Here's how the part is built. I have some questions about the finished solid (model axes, mm). A direction names the side the tool comes from. Round coordinates to 2 decimals unless told otherwise and drop trailing zeros. Loops run counter-clockwise (first coordinate to the right, second up) from the corner with the lowest first, then second, coordinate; pieces in that order, holes last. Notation, with made-up numbers: M 67.5,50 L 104.5,50 A25 cw 104.5,64 Z; hole C 63.25,-24 d11. An arc over 180 degrees is marked long. Answer as CSV lines item,"result".
```python
from build123d import *

# Parameters (mm, degrees)
SKETCH1_W           = 92.25
SKETCH1_H           = 72
SKETCH1_R           = 15
BOSS_EXTRUDE1_DEPTH = 36
BOSS_EXTRUDE2_START = -16
SKETCH1_3_R         = 36
SKETCH1_3_R_2       = 15
BOSS_EXTRUDE2_DEPTH = 16
SKETCH2_R           = 12
BOSS_EXTRUDE3_DEPTH = 28.575


with BuildPart() as part:
    # Sketch1 → Boss-Extrude1 (new body)
    with BuildSketch(Plane(origin=(0, 0, 0), x_dir=(1, 0, 0), z_dir=(0, 1, 0))):
        Rectangle(SKETCH1_W, SKETCH1_H)
        with Locations(Location((0, 0, 0), (0, 0, 270))):
            Circle(SKETCH1_R, mode=Mode.SUBTRACT)
    extrude(amount=BOSS_EXTRUDE1_DEPTH)

    # Sketch1_3 → Boss-Extrude2 (add)
    with BuildSketch(Plane(origin=(0, 0, 0), x_dir=(1, 0, 0), z_dir=(0, 1, 0)).offset(BOSS_EXTRUDE2_START)):
        with Locations(Location((0, 0, 0), (0, 0, 270))):
            Circle(SKETCH1_3_R)
        with Locations(Location((0, 0, 0), (0, 0, 270))):
            Circle(SKETCH1_3_R_2, mode=Mode.SUBTRACT)
    extrude(amount=BOSS_EXTRUDE2_DEPTH)

    # Sketch2 → Boss-Extrude3 (add)
    with BuildSketch(Plane.ZY.offset(46.125)):
        with BuildLine():
            Line((-36, 36), (36, 36))
            Line((36, 36), (36, 96))
            ThreePointArc((36, 96), (0, 132), (-36, 96))
            Line((-36, 96), (-36, 36))
        make_face()
        with Locations((0, 96)):
            Circle(SKETCH2_R, mode=Mode.SUBTRACT)
    boss_extrude3 = extrude(amount=-BOSS_EXTRUDE3_DEPTH)

    # Mirror1: Boss-Extrude3 across plane
    add(boss_extrude3.mirror(Plane(origin=(0, 0, 0), x_dir=(0, 0, 1), z_dir=(1, 0, 0))))


solid = part.part
```
1. I want a section at B-B, the plane z = 0. Please give me the cut outline in (x, y) (3 decimals), and give its area (3 significant figures).
Evaluation:
outline,"M -46.125,0 L -36,0 L -36,-16 L -15,-16 L -15,36 L -17.55,36 L -17.55,84 L -46.125,84 Z; M -46.125,108 L -17.55,108 L -17.55,132 L -46.125,132 Z; M 15,-16 L 36,-16 L 36,0 L 46.125,0 L 46.125,84 L 17.55,84 L 17.55,36 L 15,36 Z; M 17.55,108 L 46.125,108 L 46.125,132 L 17.55,132 Z"
area,"7,030 mm²"
2. I want a section at D-D, the plane x = 40.5. Please give me the cut outline in (y, z).
Evaluation:
outline,"M 0,-36 L 96,-36 A36 ccw 96,36 L 0,36 Z; hole C 96,0 d24"
3. For P1, Ø1.5, axis at x = -34, y = 98.5, coming from the +Z side; P2, Ø12, axis at x = -25, z = -18.5, coming from the +Y side; P3, Ø17.5, axis at x = -2.5, z = -7, coming from the +Y side, each with a flat end and sliding along its axis, tell me the tip position at first contact or that it passes through.
Evaluation:
P1,"stops at z = 35.96"
P2,"stops at y = 129.76"
P3,"stops at y = 36"
4. If I drill on line 1 (X direction, y = 86, z = 11.5) (3 decimals); line 2 (Y direction, x = 23.75, z = 0); line 3 (Y direction, x = -39.25, z = 0), over which ranges is the centre line in solid material (lowest first)? Write a range as [from, to].
Evaluation:
line 1,"x = [-46.125, -17.55], [17.55, 46.125]"
line 2,"y = [-16, 84], [108, 132]"
line 3,"y = [0, 84], [108, 132]"
5. Which directions (+Z, -Z, +X, -X, +Y, -Y) give clear straight access to the entire face, cutting with the end or side of a thin tool? Please do faces 1 (the flat face through (15.4, 36, -0.5)), 2 (the flat face through (-46.125, 67, -1)), 3 (the flat face through (-39, 0, -1)), 4 (the flat face through (38, 0, -1)).
Evaluation:
face 1,"+Z, -Z, +Y"
face 2,"+Z, -Z, -X, +Y, -Y"
face 3,"-X, -Y"
face 4,"+X, -Y"
6. I want a section at A-A, the plane y = 44.5. Please give me the cut outline in (x, z) (3 decimals).
Evaluation:
outline,"M -46.125,-36 L -17.55,-36 L -17.55,36 L -46.125,36 Z; M 17.55,-36 L 46.125,-36 L 46.125,36 L 17.55,36 Z"
7. I want a section at C-C, the plane y = 88. Please give me the cut outline in (x, z) (3 decimals).
Evaluation:
outline,"M -46.125,-36 L -17.55,-36 L -17.55,-8.944 L -46.125,-8.944 Z; M -46.125,8.944 L -17.55,8.944 L -17.55,36 L -46.125,36 Z; M 17.55,-36 L 46.125,-36 L 46.125,-8.944 L 17.55,-8.944 Z; M 17.55,8.944 L 46.125,8.944 L 46.125,36 L 17.55,36 Z"
8. We'd pull the mould along X, two halves only. Please class faces 5 (the flat face through (-15.5, -16, -0.5)), 6 (the cylindrical face through (10.81, -8.11, 34.34)), 7 (the flat face through (17.55, 74, -1)), 8 (the flat face through (46.125, 67, -1)): pulls with the +X half, pulls with the -X half, needs draft (parallel to the pull), parting line crosses it, or undercut.
Evaluation:
face 5,"needs draft"
face 6,"parting line crosses it"
face 7,"undercut"
face 8,"pulls with the +X half"
